Check sheet for the modelled part. Datum: model origin and axes. Units: mm. Round coordinates to 2 decimals unless told otherwise and drop trailing zeros. Loops run counter-clockwise (first coordinate to the right, second up) from the corner with the lowest first, then second, coordinate; pieces in that order, holes last. Notation, with made-up numbers: M 75,85.5 L 112,85.5 A15 cw 112,103.5 Z; hole C -1,60 d11. An arc over 180 degrees is marked long. One line per question, with ' | ' between items. Start each with the question number.
(1) Thickness scan on probe 1 along Z at (x, y) = (0, 13); probe 2 along Y at (x, z) = (-2, 465). Record the ranges inside material, lowest first. Write a range as [from, to].
(2) Go/stop test with flat-tipped pins: P1, Ø3, axis at x = -8.5, z = 109.5, coming from the +Y side; P2, Ø8, axis at x = -13, y = -6, coming from the +Z side; P3, Ø12, axis at x = -15, z = 513.5, coming from the +Y side. Record where each tip stops, or that it passes through.
(3) Section check C-C (z = 60.5). Record the boundary of the cut face in (x, y), and give its area (3 significant figures).
(4) Section check A-A (y = 0). Record the boundary of the cut face in (x, z).
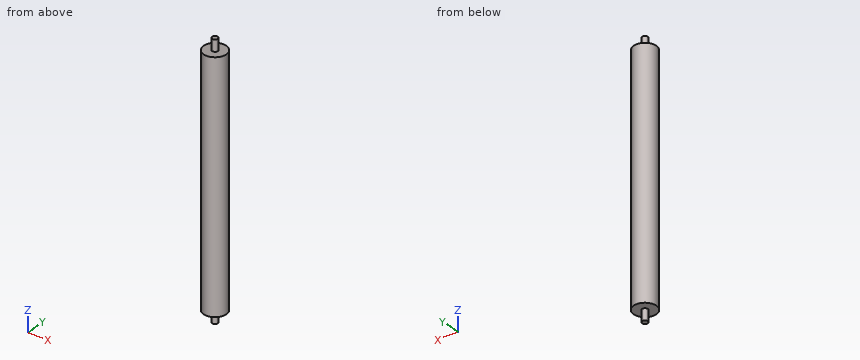
```python
from build123d import *

# Parameters (mm, degrees)
SKETCH1_R           = 25.4
BOSS_EXTRUDE1_DEPTH = 590.55
SKETCH2_OUTSIDE_W   = 171.78
SKETCH2_OUTSIDE_H   = 171.78
SKETCH2_OUTSIDE_R   = 6.361935525
CUT_EXTRUDE1_DEPTH  = 25.4
SKETCH5_OUTSIDE_W   = 171.78
SKETCH5_OUTSIDE_H   = 171.78
SKETCH5_OUTSIDE_R   = 6.377907631
CUT_EXTRUDE4_DEPTH  = 25.4
SHELL3_START        = 33.02
SHELL3_OUTLINE_R    = 17.78
SHELL3_DEPTH        = 524.51


# Read off the part's stored shape, not the designer's step: Shell3
with BuildPart() as part:
    # Sketch1 → Boss-Extrude1 (new body)
    with BuildSketch(Plane.XY):
        Circle(SKETCH1_R)
    extrude(amount=BOSS_EXTRUDE1_DEPTH)

    # Sketch2 outside → Cut-Extrude1 (cut)
    with BuildSketch(Plane.XY):
        Rectangle(SKETCH2_OUTSIDE_W, SKETCH2_OUTSIDE_H)
        Circle(SKETCH2_OUTSIDE_R, mode=Mode.SUBTRACT)
    extrude(amount=CUT_EXTRUDE1_DEPTH, mode=Mode.SUBTRACT)

    # Sketch5 outside → Cut-Extrude4 (cut)
    with BuildSketch(Plane.XY.offset(590.55)):
        Rectangle(SKETCH5_OUTSIDE_W, SKETCH5_OUTSIDE_H)
        Circle(SKETCH5_OUTSIDE_R, mode=Mode.SUBTRACT)
    extrude(amount=-CUT_EXTRUDE4_DEPTH, mode=Mode.SUBTRACT)

    # Shell3 outline → Shell3 (cut)
    with BuildSketch(Plane.XY.offset(SHELL3_START)):
        Circle(SHELL3_OUTLINE_R)
    extrude(amount=SHELL3_DEPTH, mode=Mode.SUBTRACT)


solid = part.part
```
The answers:
1) probe 1: [25.4, 33.02], [557.53, 565.15] | probe 2: [-25.32, -17.67], [17.67, 25.32]
2) P1: y = 24.42 | P2: z = 565.15 | P3: y = 23.75
3) outline: C 0,0 d50.8; hole C 0,0 d35.56 | area: 1,030 mm²
4) outline: M -25.4,25.4 L -6.36,25.4 L -6.36,0 L 6.36,0 L 6.36,25.4 L 25.4,25.4 L 25.4,565.15 L 6.38,565.15 L 6.38,590.55 L -6.38,590.55 L -6.38,565.15 L -25.4,565.15 Z; hole M -17.78,33.02 L 17.78,33.02 L 17.78,557.53 L -17.78,557.53 Z
